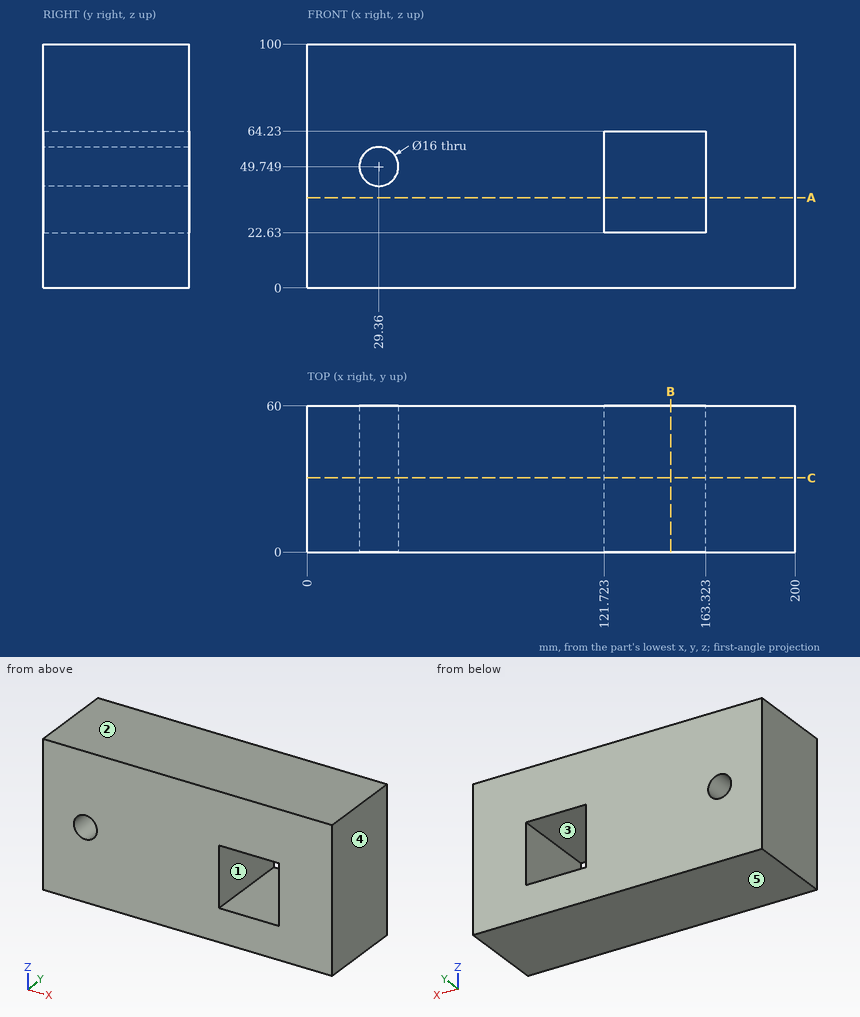
For this review, use the dimensioned drawing (mm, ordinates from the lowest corner) and the shaded views. A direction names the side the tool comes from. Give positions to 0.01 mm unless a question says otherwise; leave off trailing zeros. Write each loop counter-clockwise with the first axis right and the second up, starting at its lowest first coordinate (ties: lowest second). Pieces come first, ordered by that corner, then holes. Notation, with made-up numbers: M -37,88.5 L 19,88.5 A22 ccw 19,95.5 Z; hole C 45.5,57 d1. An arc over 180 degrees is marked long. Answer as a JSON object with one key per item and string values. Group by question number.
Item 1: Consider section B-B on x = 149. Write out the cut boundary in (y, z), plus the area to 3 significant figures.
Item 2: For probe 1 along X at (y, z) = (26, 57) (1 decimal); probe 2 along Z at (x, y) = (29, 4.5); probe 3 along X at (y, z) = (11, 53.5) (1 decimal), list the stretches that pass through material, from the lowest coordinate up. Write a range as [from, to].
Item 3: Consider section C-C on y = 30.5. Write out the cut boundary in (x, z).
Item 4: For pin 1 Ø10 at (y, z) = (39, 87.5) entering from -X, flat-tipped, find the tip position at first contact; note if it passes through.
Item 5: Consider section A-A on z = 37. Write out the cut boundary in (x, y).
Item 6: Draft analysis for pull direction X (two halves, no side actions). For the marked faces 3, 4 and 5, state which applies: +X half, -X half, draft (parallel to the pull), parting line (faces both ways), or undercut.
Item 7: Tool access review of the marked faces 1 and 2: name each direction out of +Z, -Z, +X, -X, +Y, -Y from which nothing blocks a thin tool from reaching the whole face with its end or side.
Check result:
{
 "1": {"outline": "M 0,0 L 60,0 L 60,22.63 L 0,22.63 Z; M 0,64.23 L 60,64.23 L 60,100 L 0,100 Z", "area": "3,500 mm^2"},
 "2": {"probe 1": "x = [0, 26], [32.7, 121.7], [163.3, 200]", "probe 2": "z = [0, 41.76], [57.74, 100]", "probe 3": "x = [0, 22.3], [36.4, 121.7], [163.3, 200]"},
 "3": {"outline": "M 0,0 L 200,0 L 200,100 L 0,100 Z; hole C 29.36,49.75 d16; hole M 121.72,22.63 L 163.32,22.63 L 163.32,64.23 L 121.72,64.23 Z"},
 "4": {"pin 1": "stops at x = 0"},
 "5": {"outline": "M 0,0 L 121.72,0 L 121.72,60 L 0,60 Z; M 163.32,0 L 200,0 L 200,60 L 163.32,60 Z"},
 "6": {"face 3": "undercut", "face 4": "+X half", "face 5": "draft"},
 "7": {"face 1": "+Y, -Y", "face 2": "+Z, +X, -X, +Y, -Y"}
}
